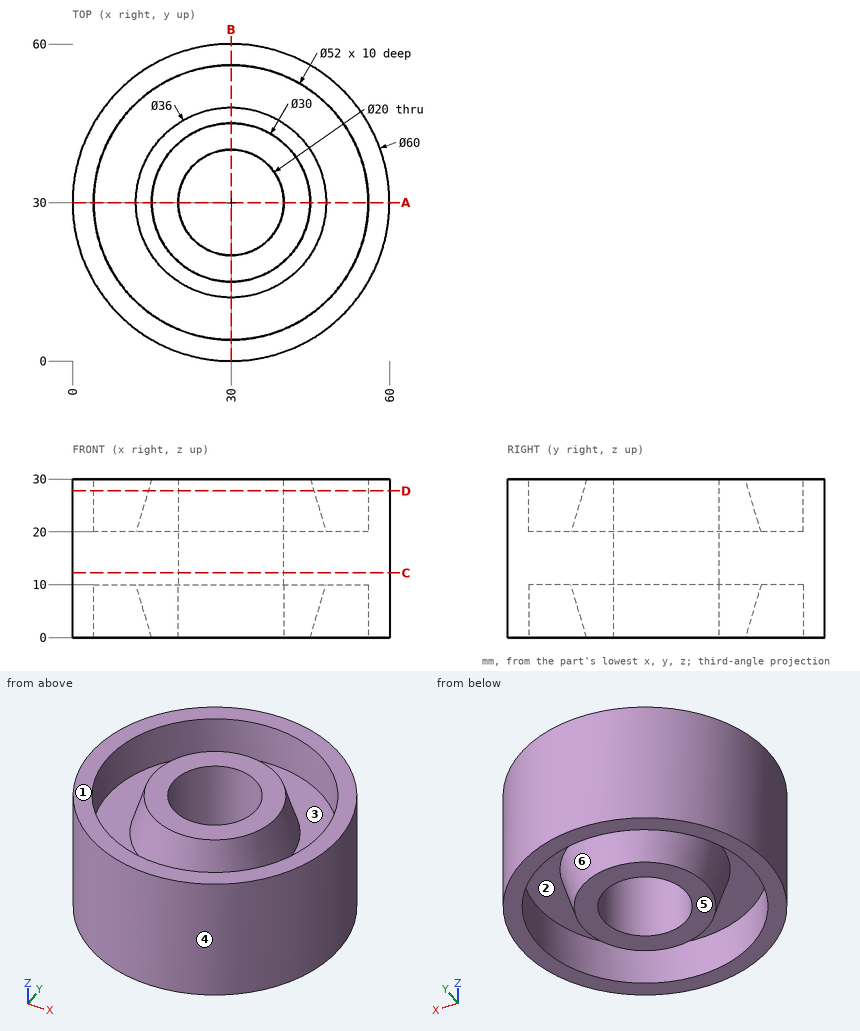
Here's the drawing with two shaded views (mm, measured from the low corner). I have some questions. A direction names the side the tool comes from. Coordinates: 2 decimals unless noted, no trailing zeros. Order: outer loops, then holes, each group sorted by start corner. A loop starts at its lowest first (then second) coordinate and runs counter-clockwise, first axis right, second up. Notation, with made-up numbers: (46.5, -7.75) - (64.5, -7.75) arc R20 cw to (64.5, 2.25) - close; hole circle Ø1 at (-7, 35). An arc over 180 degrees is marked (long way). Answer in a Markdown table with one row per item.
1. Suppose I cut it at D-D (z = 27.75). Please give me the cut outline in (x, y) (3 decimals), and give its area (3 significant figures).
Reply:
| item | result |
|---|---|
| outline | circle Ø60 at (30, 30); circle Ø31.35 at (30, 30); hole circle Ø52 at (30, 30); hole circle Ø20 at (30, 30) |
| area | 1,160 mm^2 |
2. If we mould it in two halves opening along X, with no side actions, what happens to the marked faces 4, 5 and 6? For each: pulls with the +X half, pulls with the -X half, needs draft (parallel to the pull), parting line crosses it, or undercut.
Reply:
| item | result |
|---|---|
| face 4 | parting line crosses it |
| face 5 | needs draft |
| face 6 | undercut |
3. If I drill on line 1 along Y through (x, z) = (30, 21); line 2 along Y through (x, z) = (44.5, 26.25); line 3 along X through (y, z) = (30.5, 26.5), over which ranges is the centre line in solid material (lowest first)?
Reply:
| item | result |
|---|---|
| line 1 | y = 0 to 4, 12.3 to 20, 40 to 47.7, 56 to 60 |
| line 2 | y = 3.74 to 8.42, 22.95 to 37.05, 51.58 to 56.26 |
| line 3 | x = 0 to 4, 13.96 to 20.01, 39.99 to 46.04, 56 to 60 |
4. For pin 1 (1.5 mm diameter, centred on y = 49.5, z = 15, fed in from -X); pin 2 (12 mm diameter, centred on x = 20, z = 4.5, fed in from -Y); pin 3 (8 mm diameter, centred on x = 19.5, y = 10, fed in from -Z); pin 4 (5 mm diameter, centred on x = 32.5, y = 35, fed in from -Z), each with a flat end and sliding along its axis, tell me the tip position at first contact or that it passes through.
Reply:
| item | result |
|---|---|
| pin 1 | stops at x = 6.58 |
| pin 2 | stops at y = 0.27 |
| pin 3 | stops at z = 0 |
| pin 4 | passes through |
5. For the marked faces 1, 2 and 3, which set-ups out of +Z, -Z, +X, -X, +Y, -Y let a thin tool reach every point of the face, with its end or its side?
Reply:
| item | result |
|---|---|
| face 1 | +Z, +X, -X, +Y, -Y |
| face 2 | -Z |
| face 3 | +Z |
6. Suppose I cut it at A-A (y = 30). Please give me the cut outline in (x, z), and give its area (3 significant figures).
Reply:
| item | result |
|---|---|
| outline | (0, 0) - (4, 0) - (4, 10) - (12, 10) - (15, 0) - (20, 0) - (20, 30) - (15, 30) - (12, 20) - (4, 20) - (4, 30) - (0, 30) - close; (40, 0) - (45, 0) - (48, 10) - (56, 10) - (56, 0) - (60, 0) - (60, 30) - (56, 30) - (56, 20) - (48, 20) - (45, 30) - (40, 30) - close |
| area | 820 mm^2 |
7. Suppose I cut it at C-C (z = 12.25). Please give me the cut outline in (x, y).
Reply:
| item | result |
|---|---|
| outline | circle Ø60 at (30, 30); hole circle Ø20 at (30, 30) |
